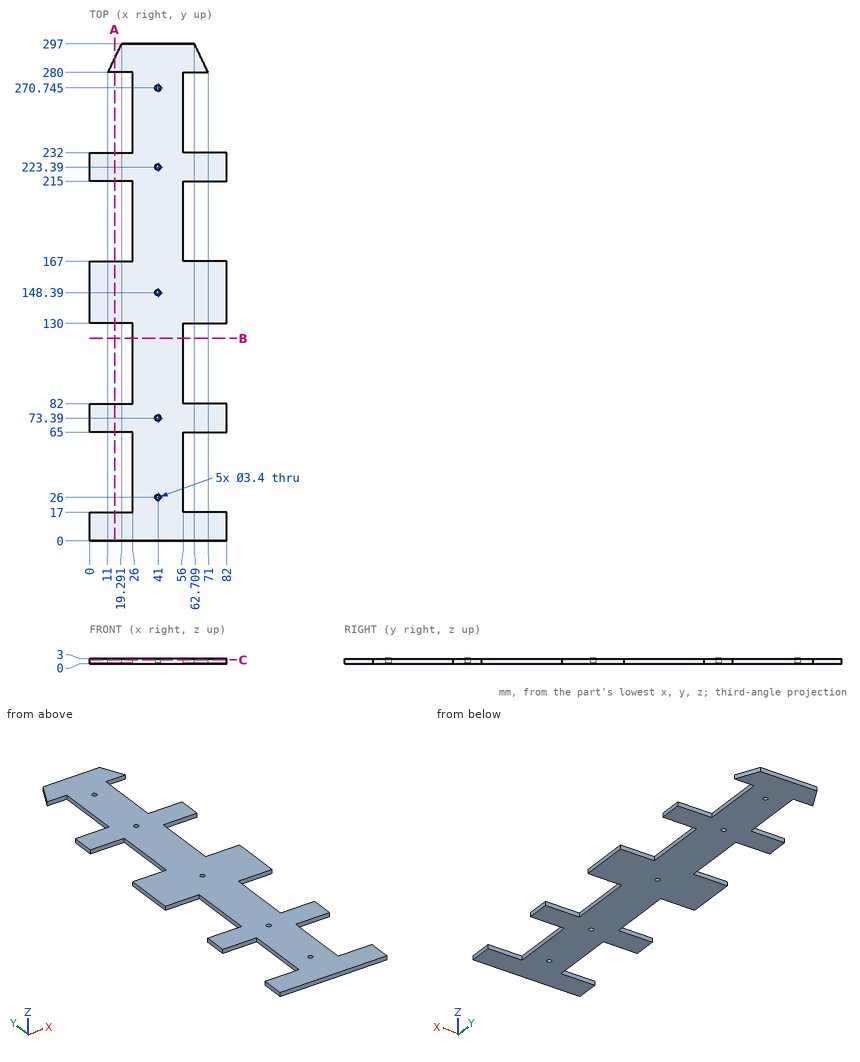
The drawing under review shows one solid part. Ordinate dimensions are in mm from its lowest x, y, z. Give positions to 0.01 mm unless a question says otherwise; leave off trailing zeros. Write each loop counter-clockwise with the first axis right and the second up, starting at its lowest first coordinate (ties: lowest second). Pieces come first, ordered by that corner, then holes. Notation, with made-up numbers: (-38.75, -1) - (-24.75, -1) arc R17 ccw to (-24.75, 22) - close; hole circle Ø3 at (60.5, -34.75). An arc over 180 degrees is marked (long way). Answer in a Markdown table with one row per item. Add a question column.
1. We need section A-A on x = 15. Write out the cut boundary in (y, z).
2. Wall thickness on line 1 along Y through (x, z) = (41, 1.3) (1 decimal); line 2 along Y through (x, z) = (20.5, 2.35); line 3 along Y through (x, z) = (67.5, 2.4) (1 decimal): over which ranges is each line inside the solid? List them lowest first. Write a range as [from, to].
3. Insertion check: P1, Ø0.9, axis at x = 63, z = 1.5, coming from the -Y side; P2, Ø0.9, axis at x = 72, z = 1.5, coming from the +Y side. Each pin has a flat end and moves straight along its axis. Give the tip position at first contact, or say it passes through.
4. We need section C-C on z = 2.4. State how many separate pieces and enclosed holes the cut face has, then the cut area to 3 significant figures.
5. We need section B-B on y = 121. Write out the cut boundary in (x, z).
Ans:
| question | item | result |
|---|---|---|
| 1 | outline | (0, 0) - (17, 0) - (17, 3) - (0, 3) - close; (65, 0) - (82, 0) - (82, 3) - (65, 3) - close; (130, 0) - (167, 0) - (167, 3) - (130, 3) - close; (215, 0) - (232, 0) - (232, 3) - (215, 3) - close; (280, 0) - (288.2, 0) - (288.2, 3) - (280, 3) - close |
| 2 | line 1 | y = [0, 24.3], [27.7, 71.7], [75.1, 146.7], [150.1, 221.7], [225.1, 269], [272.4, 297] |
| 2 | line 2 | y = [0, 17], [65, 82], [130, 167], [215, 232], [280, 297] |
| 2 | line 3 | y = [0, 17], [65, 82], [130, 167], [215, 232], [280, 287.2] |
| 3 | P1 | stops at y = 0 |
| 3 | P2 | stops at y = 232 |
| 4 | separate pieces | 1 |
| 4 | enclosed holes | 5 |
| 4 | area | 13,800 mm^2 |
| 5 | outline | (26, 0) - (56, 0) - (56, 3) - (26, 3) - close |
